Design review of the part built by this model. Coordinates are the model's own, in mm. Face numbers are marked on the shaded views. A direction names the side the tool comes from. Give positions to 0.01 mm unless a question says otherwise; leave off trailing zeros. Order: outer loops, then holes, each group sorted by start corner. A loop starts at its lowest first (then second) coordinate and runs counter-clockwise, first axis right, second up. Notation, with made-up numbers: (-6.5, 77.25) -> (0.5, 77.25) arc R17 ccw to (0.5, 101.25) -> close; hole circle Ø10 at (1, 29). An arc over 180 degrees is marked (long way). Answer in a Markdown table with one row per item. Add a question column.
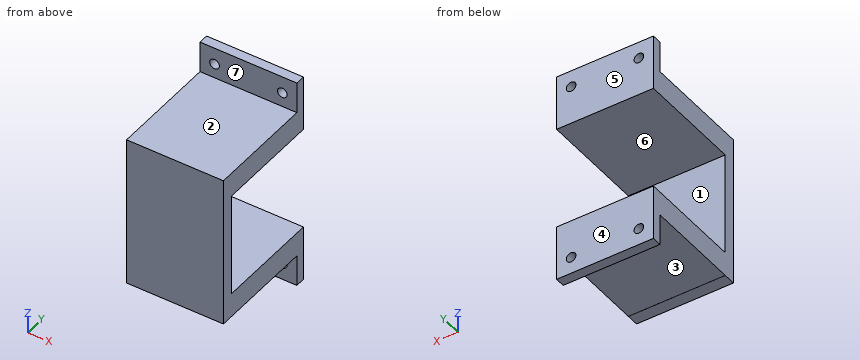
Autodesk Inventor part; units mm, degrees
ref_plane "YZ Plane" through (0, 0, 0) normal (1, 0, 0) x (0, 1, 0)
ref_plane "XZ Plane" through (0, 0, 0) normal (0, 1, 0) x (-1, 0, 0)
sketch "Sketch1" plane through (0, 0, 0) normal (0, 1, 0) x (-1, 0, 0)
  line L0 (20, 31.455) -> (-20, 31.455)
  line L1 (-20, 31.455) -> (-20, -31.455)
  line L2 (-20, -31.455) -> (20, -31.455)
  line L3 (20, -31.455) -> (20, 31.455)
  point P0 (0, 0)
  point P1 (0, 31.455)
  point P2 (20, 0)
  dimension "d0" = 40
  dimension "d1" = 62.91
extrude "Extrusion1" add sketch "Sketch1" along normal blind 5
sketch "Sketch2" plane through (0, 5, 0) normal (0, 1, 0) x (1, 0, 0)
  line L0 (-20, -31.455) -> (20, -31.455)
  line L1 (20, -31.455) -> (20, 31.455)
  line L2 (-20, -31.455) -> (20, -31.455)
  line L3 (20, -31.455) -> (20, -21.455)
  line L4 (20, -21.455) -> (-20, -21.455)
  line L5 (-20, -21.455) -> (-20, -31.455)
  line L6 (-20, 31.4422) -> (20, 31.4422)
  line L7 (20, 31.4422) -> (20, 21.4422)
  line L8 (20, 21.4422) -> (-20, 21.4422)
  line L9 (-20, 21.4422) -> (-20, 31.4422)
  line L10 (20, 31.455) -> (-20, 31.455)
  point P0 (0, 0)
  dimension "d4" = 10
  dimension "d5" = 10
  dimension "d6" = 0.0128
  dimension "d7" = 40
extrude "Extrusion2" add sketch "Sketch2" along normal blind 43.91
sketch "Sketch3" plane through (20, 5, -31.4422) normal (0, 0, -1) x (-1, 0, 0)
  line L0 (40, -5) -> (40, 43.91)
  line L1 (0, -5) -> (0, 43.91)
  line L2 (40, 43.91) -> (0, 43.91)
  line L3 (0, 43.91) -> (0, 39.91)
  line L4 (0, 39.91) -> (40, 39.91)
  line L5 (40, 39.91) -> (40, 43.91)
  point P0 (20, -5)
  dimension "d10" = 4
extrude "Extrusion3" add sketch "Sketch3" along normal blind 13
sketch "Sketch5" plane through (-20, 44.91, -31.4422) normal (0, -1, 0) x (1, 0, 0)
  circle A0 centre (34, -6.0128) radius 2
  circle A1 centre (6, -6.0128) radius 2
  line L0 (40, 0) -> (40, -13)
  line L1 (0, 0) -> (0, -13)
  line L2 (40, -0.0128) -> (0, -0.0128)
  point P0 (20, 31.4422)
  dimension "d17" = 4
  dimension "d18" = 4
  dimension "d19" = 6
  dimension "d20" = 6
  dimension "d21" = 6
extrude "Extrusion5" cut sketch "Sketch5" against normal through all
mirror "Mirror1" about plane through (0, 0, 0) normal (0, 0, 1) of "Extrusion3", "Extrusion5"
properties part number "BaseClamp"
1) Clearance check with flat-ended pins moving along their axes: P1, Ø5.5, axis at x = -1.5, y = 2.5, coming from the -Z side (3 decimals); P2, Ø6, axis at x = 9, z = 1, coming from the +Y side; P3, Ø3.5, axis at x = -14, z = -37.455, coming from the -Y side; P4, Ø5, axis at x = -5, y = 18, coming from the +Z side (3 decimals). State where each tip first meets the part, or that it passes through.
2) Add section B-B, the plane y = 35.5. Write out the cut boundary in (x, z) (3 decimals), and give its area (3 significant figures).
3) Mouldability with a two-part tool opening along Z and no side actions: class the marked faces 1, 2, 3 and 4 as +Z half, -Z half, draft (parallel to the pull), parting line (faces both ways), or undercut.
4) Add section C-C, the plane x = -8. Write out the cut boundary in (y, z) (3 decimals), and give its area (3 significant figures).
5) Machinability: for the marked faces 5, 6 and 7, which of the approach directions +Z, -Z, +X, -X, +Y, -Y give a long, thin tool a straight path to every point of the face, cutting with its end or side? Answer none if there is none.
6) For L1, parallel to Z at x = 14, y = 46 (3 decimals); L2, parallel to Z at x = 12, y = 31.5 (3 decimals); L3, parallel to Z at x = -0.5, y = 46.5 (3 decimals), list the stretches that pass through material, from the lowest coordinate up.
7) Add section A-A, the plane x = 14. Write out the cut boundary in (y, z) (3 decimals), and give its area (3 significant figures).
8) Add section D-D, the plane z = -13.5. Write out the cut boundary in (x, y).
Verdict:
| question | item | result |
|---|---|---|
| 1 | P1 | stops at z = -31.455 |
| 1 | P2 | stops at y = 5 |
| 1 | P3 | passes through |
| 1 | P4 | stops at z = 31.455 |
| 2 | outline | (-20, -31.442) -> (20, -31.442) -> (20, -21.442) -> (-20, -21.442) -> close; (-20, 21.455) -> (20, 21.455) -> (20, 31.455) -> (-20, 31.455) -> close |
| 2 | area | 800 mm2 |
| 3 | face 1 | undercut |
| 3 | face 2 | +Z half |
| 3 | face 3 | -Z half |
| 3 | face 4 | draft |
| 4 | outline | (0, -31.455) -> (5, -31.455) -> (5, -31.442) -> (44.91, -31.442) -> (44.91, -44.442) -> (48.91, -44.442) -> (48.91, -21.442) -> (5, -21.442) -> (5, 21.455) -> (48.91, 21.455) -> (48.91, 44.442) -> (44.91, 44.442) -> (44.91, 31.455) -> (0, 31.455) -> close |
| 4 | area | 1,300 mm2 |
| 5 | face 5 | +Z, -Z, +X, -X, +Y |
| 5 | face 6 | +X, -X, +Y |
| 5 | face 7 | +Z, +X, -X, -Y |
| 6 | L1 | z = -44.442 to -39.455, -35.455 to -21.442, 21.455 to 35.455, 39.455 to 44.442 |
| 6 | L2 | z = -31.442 to -21.442, 21.455 to 31.455 |
| 6 | L3 | z = -44.442 to -21.442, 21.455 to 44.442 |
| 7 | outline | (0, -31.455) -> (5, -31.455) -> (5, -31.442) -> (44.91, -31.442) -> (44.91, -35.455) -> (48.91, -35.455) -> (48.91, -21.442) -> (5, -21.442) -> (5, 21.455) -> (48.91, 21.455) -> (48.91, 35.455) -> (44.91, 35.455) -> (44.91, 31.455) -> (0, 31.455) -> close; (44.91, -44.442) -> (48.91, -44.442) -> (48.91, -39.455) -> (44.91, -39.455) -> close; (44.91, 39.455) -> (48.91, 39.455) -> (48.91, 44.442) -> (44.91, 44.442) -> close |
| 7 | area | 1,260 mm2 |
| 8 | outline | (-20, 0) -> (20, 0) -> (20, 5) -> (-20, 5) -> close |
